Check sheet for the modelled part. Datum: model origin and axes. Units: mm. Face numbers are marked on the shaded views. A direction names the side the tool comes from. Give positions to 0.01 mm unless a question says otherwise; leave off trailing zeros. Order: outer loops, then holes, each group sorted by start corner. A loop starts at its lowest first (then second) coordinate and runs counter-clockwise, first axis right, second up.
```python
from build123d import *

# Parameters (mm, degrees)
F0_W      = 63.5
F0_H      = 63.5
F1_DEPTH  = 12.7
F3_W      = 63.5
F3_H      = 12.7
F4_DEPTH  = 12.7
F5_DEPTH  = 12.7
F6_W      = 31.75
F6_H      = 7.874
F7_DEPTH  = 12.701
F8_W      = 12.7
F8_H      = 63.5
F9_DEPTH  = 19.05
F10_W     = 38.1
F10_H     = 6.35
F11_DEPTH = 25.4
F12_R     = 6.7437
F13_DEPTH = 31.751
F14_R     = 14.2875
F15_DEPTH = 9.2456


with BuildPart() as f1:
    # F0 (on Top) → F1 (new body)
    with BuildSketch(Plane.XY):
        with Locations((31.75, 32.281832)):
            Rectangle(F0_W, F0_H)
    extrude(amount=F1_DEPTH)

    # F3 (on face) → F4 (join)
    with BuildSketch(Plane(origin=(0, 0, 0), x_dir=(0, -1, 0), z_dir=(-1, 0, 0))):
        with Locations((-32.281832, 6.35)):
            Rectangle(F3_W, F3_H)
    extrude(amount=F4_DEPTH)

    # F2 (on Right) → F5 (join)
    with BuildSketch(Plane.YZ):
        with BuildLine():
            Line((51.331832, 47.752), (13.231832, 47.752))
            ThreePointArc((13.231832, 47.752), (4.251576, 44.032256), (0.531832, 35.052))
            Line((0.531832, 35.052), (0.531832, 12.7))
            Line((0.531832, 12.7), (64.031832, 12.7))
            Line((64.031832, 12.7), (64.031832, 35.052))
            ThreePointArc((64.031832, 35.052), (60.312088, 44.032256), (51.331832, 47.752))
        make_face()
        with BuildLine():
            ThreePointArc((13.231832, 27.178), (5.357832, 35.052), (13.231832, 42.926))
            Line((13.231832, 42.926), (51.331832, 42.926))
            ThreePointArc((51.331832, 42.926), (59.205832, 35.052), (51.331832, 27.178))
            Line((51.331832, 27.178), (13.231832, 27.178))
        make_face(mode=Mode.SUBTRACT)
    extrude(amount=-F5_DEPTH)

    # F6 (on face) → F7 (cut, through all)
    with BuildSketch(Plane.XY.offset(12.7)):
        with Locations((31.623, 4.468832)):
            Rectangle(F6_W, F6_H)
        with Locations((31.623, 60.094832)):
            Rectangle(F6_W, F6_H)
    extrude(amount=-F7_DEPTH, mode=Mode.SUBTRACT)

    # F8 (on face) → F9 (join)
    with BuildSketch(Plane(origin=(0, 0, 0), x_dir=(1, 0, 0), z_dir=(0, 0, -1))):
        with Locations((57.15, -32.281832)):
            Rectangle(F8_W, F8_H)
    extrude(amount=F9_DEPTH)

    # F10 (on face) → F11 (cut)
    with BuildSketch(Plane.YZ.offset(63.5)):
        with Locations((32.281832, -15.875)):
            Rectangle(F10_W, F10_H)
    extrude(amount=-F11_DEPTH, mode=Mode.SUBTRACT)

    # F12 (on face) → F13 (cut, through all)
    with BuildSketch(Plane.XY.offset(12.7)):
        with Locations((31.75, 32.281832)):
            Circle(F12_R)
    extrude(amount=-F13_DEPTH, mode=Mode.SUBTRACT)

    # F14 (on face) → F15 (cut)
    with BuildSketch(Plane.XY.offset(12.7)):
        with Locations((31.75, 32.281832)):
            Circle(F14_R)
    extrude(amount=-F15_DEPTH, mode=Mode.SUBTRACT)


solid = f1.part
```
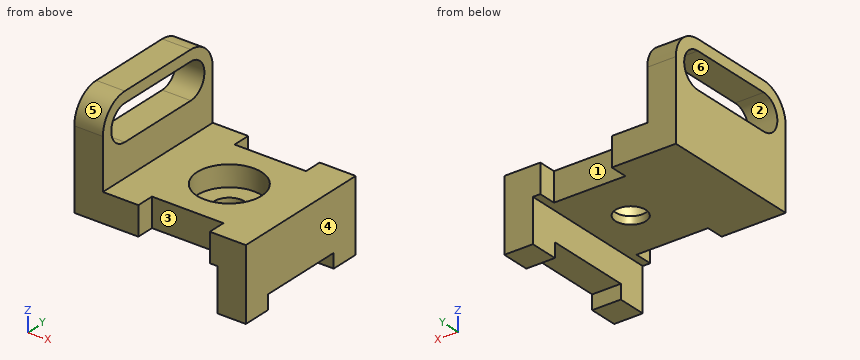
(1) Thickness scan on L1, parallel to Y at x = 31.75, z = 6.25; L2, parallel to Y at x = 31, z = 10; L3, parallel to Z at x = -3, y = 15. Record the ranges inside material, lowest first.
(2) Tool access check on the marked faces 1, 2 and 3. Record the directions out of +Z, -Z, +X, -X, +Y, -Y that give a thin tool (end or side, any length) a straight path to the whole face; none if there is none.
(3) Sectioned sample at C-C (y = 24). Enter the section's corners in (x, z).
(4) Release check for a two-part mould opening along Z. For the marked faces 4, 5 and 6 record: released by +Z, released by -Z, zero draft, split by the parting line, or undercut.
(5) Go/stop test with flat-tipped pins: P1, Ø15.5, axis at x = 31.75, y = 32.28, coming from the +Z side; P2, Ø14, axis at x = -6.5, y = 23.5, coming from the -Z side; P3, Ø15, axis at y = 34.5, z = -11.5, coming from the -X side; P4, Ø8, axis at x = 44, z = 20.5, coming from the -Y side. Record where each tip stops, or that it passes through.
(6) Sectioned sample at A-A (x = 31.75). Enter the section's corners in (y, z), plus the area to 3 significant figures.
(7) Sectioned sample at B-B (x = -4). Enter the section's corners in (y, z), plus the area to 3 significant figures.
(8) Sectioned sample at D-D (x = 21.5). Enter the section's corners in (y, z), plus the area to 3 significant figures.
Values follow:
1. L1: y = 8.41 to 17.99, 46.57 to 56.16
1. L2: y = 8.41 to 18.01, 46.55 to 56.16
1. L3: z = 0 to 27.18, 42.93 to 47.75
2. face 1: +Z, -Z, +Y
2. face 2: +X, -X
2. face 3: +Z, -Z, -Y
3. outline: (-12.7, 0) - (50.8, 0) - (50.8, -12.7) - (63.5, -12.7) - (63.5, 12.7) - (43.39, 12.7) - (43.39, 3.45) - (20.11, 3.45) - (20.11, 12.7) - (0, 12.7) - (0, 27.18) - (-12.7, 27.18) - close; (-12.7, 42.93) - (0, 42.93) - (0, 47.75) - (-12.7, 47.75) - close
4. face 4: zero draft
4. face 5: released by +Z
4. face 6: undercut
5. P1: stops at z = 3.45
5. P2: stops at z = 0
5. P3: stops at x = 50.8
5. P4: passes through
6. outline: (8.41, 0) - (25.54, 0) - (25.54, 3.45) - (17.99, 3.45) - (17.99, 12.7) - (8.41, 12.7) - close; (39.03, 0) - (56.16, 0) - (56.16, 12.7) - (46.57, 12.7) - (46.57, 3.45) - (39.03, 3.45) - close
6. area: 296 mm2
7. outline: (0.53, 0) - (64.03, 0) - (64.03, 35.05) arc R12.7 ccw to (51.33, 47.75) - (13.23, 47.75) arc R12.7 ccw to (0.53, 35.05) - close; hole (13.23, 27.18) - (51.33, 27.18) arc R7.87 ccw to (51.33, 42.93) - (13.23, 42.93) arc R7.87 ccw to start
7. area: 2,170 mm2
8. outline: (8.41, 0) - (56.16, 0) - (56.16, 12.7) - (42.24, 12.7) - (42.24, 3.45) - (22.33, 3.45) - (22.33, 12.7) - (8.41, 12.7) - close
8. area: 422 mm2
